Input: part model. Units: mm. Frame: model coordinates. A direction names the side the tool comes from. Coordinates: 2 decimals unless noted, no trailing zeros. Write each loop counter-clockwise with the first axis right and the second up, starting at its lowest first coordinate (ties: lowest second). Pieces come first, ordered by that corner, then holes.
1) Section query A-A (y = 1.45). Output: boundary loops of the cut face in (x, z).
2) Set-up query: faces 1 (the flat face through (0, 1, 51.268)), 2 (the flat face through (0, 1, -11.232)), 3 (the flat face through (0, 1, -13.232)), 4 (the flat face through (-35, 1, 19)). Return all of +Z, -Z, +X, -X, +Y, -Y with unobstructed straight access to the full face (end or side cutting, diameter ignored); none if empty.
3) Section query C-C (z = -3). Output: boundary loops of the cut face in (x, y), then the cut area to 3 significant figures.
4) Draft query along Z for faces 5 (the flat face through (0, 1, 49.268)), 6 (the cylindrical face through (-34, 2, 51)), 7 (the cylindrical face through (-35.645, 3.986, -14.08)). Return one class per face: pulls with the +Z half, pulls with the -Z half, needs draft (parallel to the pull), parting line crosses it, or undercut.
5) Line query: L1, parallel to Z at x = 3.5, y = 0.95; L2, parallel to X at y = 2.2, z = 17; L3, parallel to Y at x = 3, z = 46.5. Output: solid intervals per line, ascending.
6) Section query B-B (x = 30). Output: boundary loops of the cut face in (y, z), then the cut area to 3 significant figures.
7) Pin query (flat end, axial travel): pin 1 Ø0.9 at (y, z) = (2, 22.5) entering from -X; pin 2 Ø20.5 at (x, z) = (-7, 14) entering from -Y; pin 3 Ø2.5 at (x, y) = (12, 1.5) entering from -Z. Return the tip coordinate at first contact, or that it passes through.
from build123d import *

# Parameters (mm, degrees)
CROQUIS1_W              = 70
CROQUIS1_H              = 64.5
SALIENTE_EXTRUIR1_DEPTH = 3
REDONDEO1_R             = 2
VACIADO2_START          = -33
VACIADO2_OUTLINE_W      = 3
VACIADO2_OUTLINE_H      = 60.5
VACIADO2_DEPTH          = 66
SALIENTE_EXTRUIR2_DEPTH = 2


# Read off the part's stored shape, not the designer's step: Vaciado2
with BuildPart() as part:
    # Croquis1 → Saliente-Extruir1 (new body)
    with BuildSketch(Plane(origin=(0, 0, 0), x_dir=(1, 0, 0), z_dir=(0, 1, 0))):
        with Locations((0, -19.018292683)):
            Rectangle(CROQUIS1_W, CROQUIS1_H)
    extrude(amount=SALIENTE_EXTRUIR1_DEPTH)

    # Redondeo1
    redondeo1_edges = [part.edges().sort_by_distance(p)[0] for p in [
        (-35, 1.5, -13.231707317),
        (35, 1.5, -13.231707317),
        (35, 1.5, 51.268292683),
        (-35, 1.5, 51.268292683),
    ]]
    fillet(redondeo1_edges, radius=REDONDEO1_R)

    # Vaciado2 outline → Vaciado2 (cut)
    with BuildSketch(Plane.YZ.offset(VACIADO2_START)):
        with Locations((1.5, 19.018292683)):
            Rectangle(VACIADO2_OUTLINE_W, VACIADO2_OUTLINE_H)
    extrude(amount=VACIADO2_DEPTH, mode=Mode.SUBTRACT)

    # Croquis4 → Saliente-Extruir2 (add)
    with BuildSketch(Plane(origin=(0, 3, 0), x_dir=(1, 0, 0), z_dir=(0, 1, 0))):
        with BuildLine():
            Line((33.5, -53.018292683), (-33.5, -53.018292683))
            ThreePointArc((-33.5, -53.018292683), (-35.621320344, -52.139613026), (-36.5, -50.018292683))
            Line((-36.5, -50.018292683), (-36.5, 11.981707317))
            ThreePointArc((-36.5, 11.981707317), (-35.621320344, 14.103027661), (-33.5, 14.981707317))
            Line((-33.5, 14.981707317), (33.5, 14.981707317))
            ThreePointArc((33.5, 14.981707317), (35.621320344, 14.103027661), (36.5, 11.981707317))
            Line((36.5, 11.981707317), (36.5, -50.018292683))
            ThreePointArc((36.5, -50.018292683), (35.621320344, -52.139613026), (33.5, -53.018292683))
        make_face()
    extrude(amount=SALIENTE_EXTRUIR2_DEPTH)


solid = part.part
Answer:
1. outline: (-35, -11.23) arc R2 ccw to (-33, -13.23) - (33, -13.23) arc R2 ccw to (35, -11.23) - (35, 49.27) arc R2 ccw to (33, 51.27) - (-33, 51.27) arc R2 ccw to (-35, 49.27) - close; hole (-33, -11.23) - (33, -11.23) - (33, 49.27) - (-33, 49.27) - close
2. face 1: +Z, +X, -X, -Y
2. face 2: -Y
2. face 3: -Z, +X, -X, -Y
2. face 4: +Z, -Z, -X, -Y
3. outline: (-36.5, 3) - (-35, 3) - (-35, 0) - (-33, 0) - (-33, 3) - (33, 3) - (33, 0) - (35, 0) - (35, 3) - (36.5, 3) - (36.5, 5) - (-36.5, 5) - close
3. area: 158 mm2
4. face 5: undercut
4. face 6: pulls with the +Z half
4. face 7: pulls with the -Z half
5. L1: z = -13.23 to -11.23, 49.27 to 51.27
5. L2: x = -35 to -33, 33 to 35
5. L3: y = 3 to 5
6. outline: (0, -13.23) - (3, -13.23) - (3, -14.98) - (5, -14.98) - (5, 53.02) - (3, 53.02) - (3, 51.27) - (0, 51.27) - (0, 49.27) - (3, 49.27) - (3, -11.23) - (0, -11.23) - close
6. area: 148 mm2
7. pin 1: stops at x = -35
7. pin 2: stops at y = 3
7. pin 3: stops at z = -13.23
